Verification items for the finished model (mm, model axes). A direction names the side the tool comes from. Round coordinates to 2 decimals unless told otherwise and drop trailing zeros. Order: outer loops, then holes, each group sorted by start corner. A loop starts at its lowest first (then second) coordinate and runs counter-clockwise, first axis right, second up. Notation, with made-up numbers: M 85.5,12 L 125.5,12 A16 ccw 125.5,32 Z; hole C -1,-0.5 d4. An arc over 180 degrees is marked long. Use CSV: the item, a comma, the result in double quotes. Start each with the question number.
Q1. Gauge pin test, flat ends, axial feed: pin 1 Ø5 at (y, z) = (11, -125.5) entering from +X; pin 2 Ø1.5 at (x, z) = (6, -136.5) entering from +Y; pin 3 Ø2 at (y, z) = (-7, 38.5) entering from +X; pin 4 Ø3 at (x, y) = (0.5, 13) entering from +Z. Record the tip position at first contact, or that the pin passes through.
Q2. Sectioned sample at B-B (y = 0). Enter the section's corners in (x, z) (3 decimals).
Q3. Set-up check for faces 1 (the face through (0, 11.818, 38)), 2 (the face through (0, -1, -200)), 3 (the face through (0.385, -9.522, 38.198)): record each of +Z, -Z, +X, -X, +Y, -Y from which the full face is reachable in a straight line by a thin tool's end or side.
Q4. Sectioned sample at A-A (x = 0). Enter the section's corners in (y, z) (3 decimals), and give its area (3 significant figures).
Q5. Scan lines: line 1 (Y direction, x = -1, z = -11.5); line 2 (Z direction, x = 9.5, y = 1.5); line 3 (X direction, y = 13.5, z = -121). Record each from-to range of solid material in increasing order.
Q6. Sectioned sample at C-C (z = -61.5). Enter the section's corners in (x, y) (3 decimals).
```python
from build123d import *

# Parameters (mm, degrees)
BOSS_EXTRUDE1_DEPTH = 77.48
BOSS_EXTRUDE2_DEPTH = 200


with BuildPart() as part:
    # Sketch1 → Boss-Extrude1 (new body)
    with BuildSketch(Plane.XY):
        with BuildLine():
            Line((-2.38, 11.818027958), (2.38, 11.818027958))
            Line((2.38, 11.818027958), (2.38, 9.228027958))
            ThreePointArc((2.38, 9.228027958), (0, -9.53), (-2.38, 9.228027958))
            Line((-2.38, 9.228027958), (-2.38, 11.818027958))
        make_face()
    extrude(amount=BOSS_EXTRUDE1_DEPTH)

    # Sketch2 → Boss-Extrude2 (add)
    with BuildSketch(Plane(origin=(0, 0, 0), x_dir=(-1, 0, 0), z_dir=(0, 0, -1))):
        with BuildLine():
            Line((-2.38, 15.557201527), (2.38, 15.557201527))
            Line((2.38, 15.557201527), (2.38, 10.857201527))
            ThreePointArc((2.38, 10.857201527), (0, -11.115), (-2.38, 10.857201527))
            Line((-2.38, 10.857201527), (-2.38, 15.557201527))
        make_face()
    extrude(amount=BOSS_EXTRUDE2_DEPTH)


solid = part.part
```
Verdict:
1,pin 1,"stops at x = 7.16"
1,pin 2,"stops at y = 9.8"
1,pin 3,"stops at x = 7.4"
1,pin 4,"stops at z = 77.48"
2,outline,"M -11.115,-200 L 11.115,-200 L 11.115,0 L 9.53,0 L 9.53,77.48 L -9.53,77.48 L -9.53,0 L -11.115,0 Z"
3,face 1,"+Z, +X, -X, +Y"
3,face 2,"-Z, +X, -X, +Y, -Y"
3,face 3,"+Z"
4,outline,"M -11.115,-200 L 15.557,-200 L 15.557,0 L 11.818,0 L 11.818,77.48 L -9.53,77.48 L -9.53,0 L -11.115,0 Z"
4,area,"6,990 mm²"
5,line 1,"y = -11.07 to 15.56"
5,line 2,"z = -200 to 0"
5,line 3,"x = -2.38 to 2.38"
6,outline,"M -2.38,10.857 A11.115 ccw long 2.38,10.857 L 2.38,15.557 L -2.38,15.557 Z"
